CAD build for the part. Positions are in the model's coordinates, mm. Give positions to 0.01 mm unless a question says otherwise; leave off trailing zeros. Loops run counter-clockwise (first coordinate to the right, second up) from the corner with the lowest first, then second, coordinate; pieces in that order, holes last. Notation, with made-up numbers: (49.25, 5) - (70.25, 5) arc R25 ccw to (70.25, 35) - close; hole circle Ø9 at (-28, 86). An arc over 180 degrees is marked (long way). Return JSON: item names as keys, results as strings.
from build123d import *

# Parameters (mm, degrees)
F0_R     = 1.905
F0_R_2   = 6.35
F1_DEPTH = 2.54


with BuildPart() as f1:
    # F0 (on Top) → F1 (new body)
    with BuildSketch(Plane.XY):
        Polygon((-127, -177.8), (177.8, -177.8), (177.8, 190.5), (-177.8, 190.5), (-177.8, -127), (-127, -127), align=None)
        with Locations((-165.1, 0)):
            Circle(F0_R, mode=Mode.SUBTRACT)
        with Locations((0, -165.1)):
            Circle(F0_R, mode=Mode.SUBTRACT)
        with Locations((165.1, -165.1)):
            Circle(F0_R, mode=Mode.SUBTRACT)
        with Locations((165.1, 0)):
            Circle(F0_R, mode=Mode.SUBTRACT)
        with Locations((-165.1, 165.1)):
            Circle(F0_R, mode=Mode.SUBTRACT)
        with Locations((-82.55, 171.45)):
            Circle(F0_R_2, mode=Mode.SUBTRACT)
        with Locations((0, 165.1)):
            Circle(F0_R, mode=Mode.SUBTRACT)
        with Locations((82.55, 171.45)):
            Circle(F0_R_2, mode=Mode.SUBTRACT)
        with Locations((165.1, 165.1)):
            Circle(F0_R, mode=Mode.SUBTRACT)
    extrude(amount=F1_DEPTH)


solid = f1.part
1. Pull direction Y, two halves, no side cores. Call faces 1 (the face through (-87.23, 175.74, 1.25)), 2 (the face through (-2, 9, 2.54)), 3 (the face through (77.87, 175.74, 1.25)): +Y half, -Y half, draft (parallel to the pull), parting line (faces both ways), or undercut.
Values follow:
{"face 1": "undercut", "face 2": "draft", "face 3": "undercut"}
2. Drop flat-ended pins along their axis: P1, Ø0.8, axis at y = -140, z = 0.5, coming from the -X side; P2, Ø2.5, axis at x = 165.1, y = 0, coming from the -Z side; P3, Ø8, axis at x = -54, y = -101, coming from the -Z side. Give the stop position or say it passes through.
Values follow:
{"P1": "stops at x = -127", "P2": "passes through", "P3": "stops at z = 0"}
3. Cut at A-A, the plane x = -82.55. Write the cut outline in (y, z).
Values follow:
{"outline": "(-177.8, 0) - (165.1, 0) - (165.1, 2.54) - (-177.8, 2.54) - close; (177.8, 0) - (190.5, 0) - (190.5, 2.54) - (177.8, 2.54) - close"}
4. Cut at B-B, the plane y = 171.45. Write the cut outline in (x, z).
Values follow:
{"outline": "(-177.8, 0) - (-88.9, 0) - (-88.9, 2.54) - (-177.8, 2.54) - close; (-76.2, 0) - (76.2, 0) - (76.2, 2.54) - (-76.2, 2.54) - close; (88.9, 0) - (177.8, 0) - (177.8, 2.54) - (88.9, 2.54) - close"}
5. Cut at C-C, the plane z = 1. Give the number of separate pieces and of enclosed holes in the cut face, plus the area to 3 significant figures.
Values follow:
{"separate pieces": "1", "enclosed holes": "9", "area": "128,000 mm²"}
6. Drill centre lines: probe 1 along Y at (x, z) = (165.1, 1.25) (3 decimals); probe 2 along Y at (x, z) = (0, 0.65) (3 decimals); probe 3 along X at (y, z) = (-165.1, 1.35) (3 decimals). Where is each one in solid material? Low to high.
Values follow:
{"probe 1": "y = -177.8 to -167.005, -163.195 to -1.905, 1.905 to 163.195, 167.005 to 190.5", "probe 2": "y = -177.8 to -167.005, -163.195 to 163.195, 167.005 to 190.5", "probe 3": "x = -127 to -1.905, 1.905 to 163.195, 167.005 to 177.8"}
